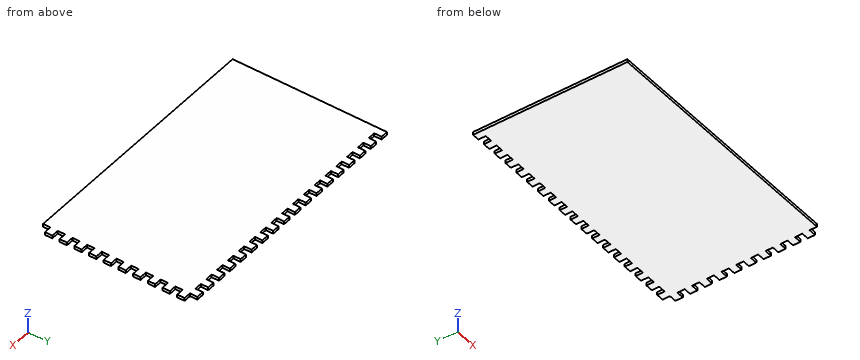
```python
from build123d import *

# Parameters (mm, degrees)
F0_W     = 5
F0_H     = 5
F1_DEPTH = 2


with BuildPart() as f1:
    # F0 (on Top) → F1 (new body)
    with BuildSketch(Plane.XY):
        Polygon((-180, -3.5), (-180, -103.5), (-5, -103.5), (-5, -98.5), (-5, -93.5), (-5, -88.5), (-5, -83.5), (-5, -78.5), (-5, -73.5), (-5, -68.5), (-5, -63.5), (-5, -58.5), (-5, -53.5), (-5, -48.5), (-5, -43.5), (-5, -38.5), (-5, -33.5), (-5, -28.5), (-5, -23.5), (-5, -18.5), (-5, -13.5), (-5, -8.5), (-5, -3.5), (-5, 1.5), (-10, 1.5), (-10, -3.5), (-15, -3.5), (-15, 1.5), (-20, 1.5), (-20, -3.5), (-25, -3.5), (-25, 1.5), (-30, 1.5), (-30, -3.5), (-35, -3.5), (-35, 1.5), (-40, 1.5), (-40, -3.5), (-45, -3.5), (-45, 1.5), (-50, 1.5), (-50, -3.5), (-55, -3.5), (-55, 1.5), (-60, 1.5), (-60, -3.5), (-65, -3.5), (-65, 1.5), (-70, 1.5), (-70, -3.5), (-75, -3.5), (-75, 1.5), (-80, 1.5), (-80, -3.5), (-85, -3.5), (-85, 1.5), (-90, 1.5), (-90, -3.5), (-95, -3.5), (-95, 1.5), (-100, 1.5), (-100, -3.5), (-105, -3.5), (-105, 1.5), (-110, 1.5), (-110, -3.5), (-115, -3.5), (-115, 1.5), (-120, 1.5), (-120, -3.5), (-125, -3.5), (-125, 1.5), (-130, 1.5), (-130, -3.5), (-135, -3.5), (-135, 1.5), (-140, 1.5), (-140, -3.5), (-145, -3.5), (-145, 1.5), (-150, 1.5), (-150, -3.5), (-155, -3.5), (-155, 1.5), (-160, 1.5), (-160, -3.5), (-165, -3.5), (-165, 1.5), (-170, 1.5), (-170, -3.5), (-175, -3.5), (-175, 1.5), (-180, 1.5), align=None)
        with Locations((-2.5, -96)):
            Rectangle(F0_W, F0_H)
        with Locations((-2.5, -86)):
            Rectangle(F0_W, F0_H)
        with Locations((-2.5, -76)):
            Rectangle(F0_W, F0_H)
        with Locations((-2.5, -66)):
            Rectangle(F0_W, F0_H)
        with Locations((-2.5, -56)):
            Rectangle(F0_W, F0_H)
        with Locations((-2.5, -46)):
            Rectangle(F0_W, F0_H)
        with Locations((-2.5, -36)):
            Rectangle(F0_W, F0_H)
        with Locations((-2.5, -26)):
            Rectangle(F0_W, F0_H)
        with Locations((-2.5, -16)):
            Rectangle(F0_W, F0_H)
        with Locations((-2.5, -6)):
            Rectangle(F0_W, F0_H)
    extrude(amount=F1_DEPTH)


solid = f1.part
```
Check sheet for the modelled part. Datum: model origin and axes. Units: mm. Round coordinates to 2 decimals unless told otherwise and drop trailing zeros. Order: outer loops, then holes, each group sorted by start corner. A loop starts at its lowest first (then second) coordinate and runs counter-clockwise, first axis right, second up.
1) Go/stop test with flat-tipped pins: pin 1 Ø0.6 at (y, z) = (0, 0.5) entering from +X; pin 2 Ø0.6 at (x, z) = (-33.5, 1.5) entering from +Y; pin 3 Ø0.6 at (x, z) = (-2.5, 1.5) entering from -Y. Record where each tip stops, or that it passes through.
2) Section check A-A (y = -80.5). Record the boundary of the cut face in (x, z), and give its area (3 significant figures).
3) Scan lines: line 1 (X direction, y = -50, z = 1.25); line 2 (Y direction, x = -30.5, z = 0.85). Record each from-to range of solid material in increasing order.
Result:
1. pin 1: stops at x = -5
1. pin 2: stops at y = -3.5
1. pin 3: stops at y = -98.5
2. outline: (-180, 0) - (-5, 0) - (-5, 2) - (-180, 2) - close
2. area: 350 mm2
3. line 1: x = -180 to -5
3. line 2: y = -103.5 to -3.5
